For this review, take the finished solid that the model builds, in its own axes (mm). A direction names the side the tool comes from. Give positions to 0.01 mm unless a question says otherwise; leave off trailing zeros. Loops run counter-clockwise (first coordinate to the right, second up) from the corner with the lowest first, then second, coordinate; pieces in that order, holes last. Notation, with made-up numbers: M 77,56 L 109,56 A32 ccw 109,83 Z; hole C 25,50 d2. An arc over 180 degrees is marked long. Use CSV: the item, a comma, the result in double quotes. Start each with the question number.
1. The part is to be moulded in two halves that separate along X. For faces 6 (the face through (0, 34.29, 3)), 7 (the face through (-12.885, 45.849, 3.757)), 8 (the face through (-11.456, 35.073, 17.737)), say which applies: pulls with the +X half, pulls with the -X half, needs draft (parallel to the pull), parting line crosses it, or undercut.
2. To check wall thickness, follow line 1 (X direction, y = 35.15, z = 12.7) (3 decimals); line 2 (X direction, y = 34.75, z = 12.7) (3 decimals); line 3 (Y direction, x = 0, z = 1.8) (1 decimal). State the ranges of each line that lie inside material, in increasing order. Write a range as [from, to].
3. Take a section at B-B, the plane y = 44. Write out the cut boundary in (x, z) (3 decimals).
4. Tool access review of faces 1 (the face through (-13.043, 43.708, 3.757)), 2 (the face through (5.543, 39.886, 5.366)), 3 (the face through (4.445, 35.5, 9.2)), 4 (the face through (-6.287, 41.765, 1.565)), 5 (the face through (10, 40, 7.62)): name each direction out of +Z, -Z, +X, -X, +Y, -Y from which nothing blocks a thin tool from reaching the whole face with its end or side.
5. Take a section at A-A, the plane x = 0. Write out the cut boundary in (y, z) (1 decimal), and give its area (3 significant figures).
6. Take a section at D-D, the plane z = 3.75. Write out the cut boundary in (x, y) (3 decimals).
7. Insertion check: P1, Ø5, axis at x = 0, y = 41.91, coming from the -Z side; P2, Ø9, axis at x = -9.5, z = 15.5, coming from the +Y side; P3, Ø3, axis at x = 12.5, y = 43, coming from the +Z side; P4, Ø1, axis at y = 36, z = 13.5, coming from the -X side. Each pin has a flat end and moves straight along its axis. Give the tip position at first contact, or say it passes through.
8. Take a section at C-C, the plane z = 11.5. State how many separate pieces and enclosed holes the cut face has, and give its area (3 significant figures).
Autodesk Inventor part; units mm, degrees
ref_plane "Work Plane1" through (-18.415, 35.8775, 0) normal (0, -1, 0) x (1, 0, 0)
ref_plane "YZ Plane" through (0, 0, 0) normal (1, 0, 0) x (0, 1, 0)
ref_plane "XZ Plane" through (0, 0, 0) normal (0, 1, 0) x (-1, 0, 0)
sketch "Sketch1" plane through (0, 0, 0) normal (0, 0, 1) x (1, 0, 0)
  circle A0 centre (0, 0) radius 47.625
  line L0 (0, 0) -> (0, 41.91)
  circle A1 centre (0, 41.91) radius 1.5875
  line L1 (-10.795, 34.29) -> (10.795, 34.29)
  circle A2 centre (0, 41.91) radius 3.175
  line L2 (-10.795, 34.29) -> (-18.415, 34.29)
  line L3 (10.795, 34.29) -> (18.415, 34.29)
  line L4 (18.415, 34.29) -> (1.6658, 44.6129)
  line L5 (-18.415, 34.29) -> (-1.6658, 44.6129)
  line L6 (-1.6658, 44.6129) -> (-3.4454, 47.5002)
  line L7 (1.6658, 44.6129) -> (3.4454, 47.5002)
  line L8 (8.1528, 40.6148) -> (11.5907, 46.193)
  line L9 (10.3151, 39.2822) -> (14.1344, 45.4792)
  line L10 (-8.1528, 40.6148) -> (-11.5907, 46.193)
  line L11 (-10.3151, 39.2822) -> (-14.1344, 45.4792)
  dimension "d0" = 95.25
  dimension "d1" = 41.91
  dimension "d2" = 3.175
  dimension "d3" = 21.59
  dimension "d4" = 7.62
  dimension "d5" = 10.795
  dimension "d6" = 6.35
  dimension "d7" = 7.62
  dimension "d8" = 7.62
  dimension "d27" = 7.62
  dimension "d28" = 2.54
  dimension "d29" = 7.62
  dimension "d30" = 2.54
extrude "Extrusion1" add sketch "Sketch1" along normal blind 3.175 contours L4 L3 L1 L0 A2 | L5 A2 L0 L1 L2 | L7 A2 L6 A0 | A2
sketch "Sketch2" plane through (0, 0, 3.175) normal (0, 0, 1) x (1, 0, 0)
  circle A0 centre (0, 41.91) radius 1.5875
  line L0 (-1.6658, 44.6129) -> (-18.415, 34.29)
  line L1 (-18.415, 34.29) -> (18.415, 34.29)
  line L2 (18.415, 34.29) -> (1.6658, 44.6129)
  line L3 (1.6658, 44.6129) -> (3.4454, 47.5002)
  arc A1 (3.4454, 47.5002) -> (-3.4454, 47.5002) centre (0, 0) ccw
  line L4 (-3.4454, 47.5002) -> (-1.6658, 44.6129)
  line L5 (-4.445, 34.29) -> (-4.445, 42.9)
  line L6 (-18.415, 34.29) -> (18.415, 34.29)
  line L7 (4.445, 34.29) -> (4.445, 42.9)
  dimension "d11" = 13.97
extrude "Extrusion2" add sketch "Sketch2" along normal blind 15.875 contours L5 L1 L0 | L7 L2 L1
sketch "Sketch3" plane through (-18.415, 34.29, 0) normal (0, -1, 0) x (1, 0, 0)
  line L0 (0, 0) -> (36.83, 0)
  line L1 (36.83, 0) -> (36.83, 19.05)
  line L2 (22.86, 19.05) -> (36.83, 19.05)
  line L3 (22.86, 3.175) -> (22.86, 19.05)
  line L4 (13.97, 3.175) -> (22.86, 3.175)
  line L5 (13.97, 3.175) -> (13.97, 19.05)
  line L6 (0, 19.05) -> (13.97, 19.05)
  line L7 (0, 0) -> (0, 19.05)
  circle A0 centre (7.62, 12.7) radius 5.08
  circle A1 centre (29.21, 12.7) radius 5.08
  point P0 (18.415, 0)
  dimension "d14" = 10.16
  dimension "d15" = 10.16
  dimension "d16" = 6.35
  dimension "d17" = 6.35
  dimension "d18" = 6.35
  dimension "d19" = 6.35
extrude "Extrusion3" cut sketch "Sketch3" against normal blind 12.7 contours A0 | A1
ref_plane "Work Plane1" through (-18.415, 35.8775, 0) normal (0, -1, 0) x (1, 0, 0)
sketch "Sketch4" plane through (-18.415, 35.8775, 0) normal (0, -1, 0) x (1, 0, 0)
  circle A0 centre (29.21, 12.7) radius 5.08
  line L0 (36.83, 0) -> (20.0808, 0)
  line L1 (20.0808, 0) -> (20.0808, 3.175)
  line L2 (22.86, 3.175) -> (20.0808, 3.175)
  line L3 (22.86, 3.175) -> (22.86, 19.05)
  line L4 (36.83, 19.05) -> (22.86, 19.05)
  line L5 (36.83, 0) -> (36.83, 19.05)
  circle A1 centre (7.62, 12.7) radius 5.08
  line L6 (16.7492, 0) -> (0, 0)
  line L7 (0, 0) -> (0, 19.05)
  line L8 (13.97, 19.05) -> (0, 19.05)
  line L9 (13.97, 3.175) -> (13.97, 19.05)
  line L10 (16.7492, 3.175) -> (13.97, 3.175)
  line L11 (16.7492, 0) -> (16.7492, 3.175)
  line L12 (36.83, 19.05) -> (22.86, 19.05)
  line L13 (36.83, 19.05) -> (22.86, 19.05)
  line L14 (22.86, 19.05) -> (22.86, 7.62)
  line L15 (22.86, 7.62) -> (36.83, 7.62)
  line L16 (36.83, 7.62) -> (36.83, 19.05)
  line L17 (0, 19.05) -> (13.97, 19.05)
  line L18 (13.97, 19.05) -> (13.97, 7.62)
  line L19 (13.97, 7.62) -> (0, 7.62)
  line L20 (0, 7.62) -> (0, 19.05)
  circle A2 centre (29.21, 12.7) radius 5.08
  circle A3 centre (7.62, 12.7) radius 5.08
  point P0 (18.415, 0)
extrude "Extrusion4" cut sketch "Sketch4" against normal blind 12.7 contours A0 | L15 L3 L4 L5 | A1 | L19 L7 L8 L9
fillet "Fillet1" radius 3.175 2 edges at (1.6658, 44.6129, 1.5875) (-1.6658, 44.6129, 1.5875)
extrude "Extrusion5" add sketch "Sketch1" along normal up to surface (7.62 mm away) contours L9 L4 L8 A0 | A0 L10 L5 L11
fillet "Fillet3" radius 3.175 2 edges at (-10.3151, 39.2822, 3.81) (10.3151, 39.2822, 3.81)
fillet "Fillet4" radius 3.175 2 edges at (-4.445, 42.9, 5.3975) (4.445, 42.9, 5.3975)
equation "\"d5\" = 0.5 * d3"
properties part number "aftPotentiometerMount" material "ABS Plastic"
Result set:
1,face 6,"needs draft"
1,face 7,"pulls with the -X half"
1,face 8,"undercut"
2,line 1,"[-17.02, -15.875], [-5.715, -4.445], [4.445, 5.715], [15.875, 17.02]"
2,line 2,"[-17.669, -15.875], [-5.715, -4.445], [4.445, 5.715], [15.875, 17.669]"
2,line 3,"[34.3, 40.3], [43.5, 47.6]"
3,outline,"M -13.223,0 L -10.239,0 L -10.239,7.62 L -13.223,7.62 Z; M -3.322,0 L 3.322,0 L 3.322,3.175 L -3.322,3.175 Z; M 10.239,0 L 13.223,0 L 13.223,7.62 L 10.239,7.62 Z"
4,face 1,"+Z, -Z, -X"
4,face 2,"+Z, +Y"
4,face 3,"+Z, +Y, -Y"
4,face 4,"+Z, -Z, +Y"
4,face 5,"+Z, +X, -X, +Y"
5,outline,"M 34.3,0 L 40.3,0 L 40.3,3.2 L 34.3,3.2 Z; M 43.5,0 L 47.6,0 L 47.6,3.2 L 43.5,3.2 Z"
5,area,"32.3 mm2"
6,outline,"M -18.415,34.29 L -4.445,34.29 L -4.445,37.485 A3.175 ccw -8.153,40.615 L -11.591,46.193 A47.625 ccw -14.134,45.479 L -11.981,41.985 A3.175 cw -13.018,37.616 Z; M 4.445,34.29 L 18.415,34.29 L 13.018,37.616 A3.175 cw 11.981,41.985 L 14.134,45.479 A47.625 ccw 11.591,46.193 L 8.153,40.615 A3.175 ccw 4.445,37.485 Z"
7,P1,"z = 0"
7,P2,"y = 35.88"
7,P3,"z = 7.62"
7,P4,"x = -16.45"
8,separate pieces,"4"
8,enclosed holes,"0"
8,area,"8.92 mm2"
